Source: CAD feature listing. Evaluate the final solid. Frame: model axes, mm. Face numbers are marked on the shaded views. A direction names the side the tool comes from. Coordinates: 2 decimals unless noted, no trailing zeros. Write each loop counter-clockwise with the first axis right and the second up, starting at its lowest first coordinate (ties: lowest second). Pieces come first, ordered by that corner, then holes. Notation, with made-up numbers: (69, -8.75) -> (96, -8.75) arc R25 cw to (96, 22.25) -> close; hole circle Ø8 at (-25.5, 53). An arc over 180 degrees is marked (long way). Write item = value, one per line.
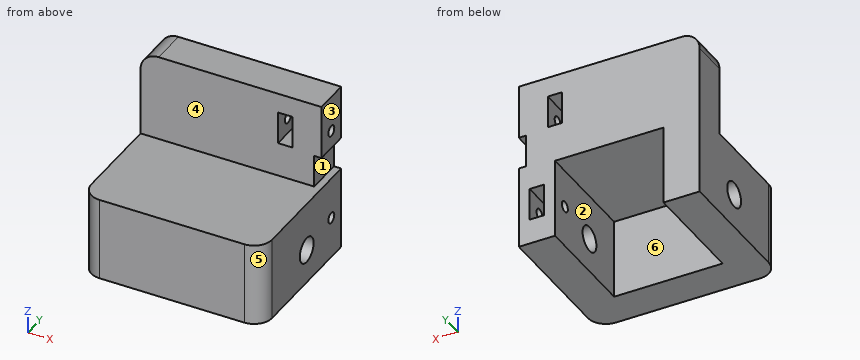
from build123d import *

# Parameters (mm, degrees)
BOSS_EXTRUDE1_DEPTH = 22
SKETCH3_W           = 10
SKETCH3_H           = 10
BOSS_EXTRUDE2_DEPTH = 25
SKETCH4_W           = 25
SKETCH4_H           = 10
BOSS_EXTRUDE3_DEPTH = 40
SKETCH5_W           = 2
SKETCH5_H           = 10
CUT_EXTRUDE4_DEPTH  = 40
BOSS_EXTRUDE4_DEPTH = 1
SKETCH7_R           = 1.5
CUT_EXTRUDE5_DEPTH  = 15
SKETCH8_W           = 4
SKETCH8_H           = 9
CUT_EXTRUDE6_DEPTH  = 15
FILLET1_R           = 5
FILLET2_R           = 5
FILLET3_R           = 5
SKETCH9_R           = 3.5
CUT_EXTRUDE7_DEPTH  = 1000
SKETCH10_W          = 4
SKETCH10_H          = 9
BOSS_EXTRUDE5_DEPTH = 15
SKETCH11_R          = 1.5
BOSS_EXTRUDE6_DEPTH = 10
SKETCH12_R          = 1.5
CUT_EXTRUDE8_DEPTH  = 19
SKETCH13_W          = 4.004831452
SKETCH13_H          = 9
CUT_EXTRUDE9_DEPTH  = 10


with BuildPart() as part:
    # Sketch1 → Boss-Extrude1 (new body)
    with BuildSketch(Plane.XY):
        Polygon((0, 30), (-10, 30), (-10, -10), (40, -10), (40, 30), (30, 30), (30, 0), (0, 0), align=None)
    extrude(amount=BOSS_EXTRUDE1_DEPTH)

    # Sketch3 → Boss-Extrude2 (add)
    with BuildSketch(Plane.XY.offset(22)):
        with Locations((-5, 25)):
            Rectangle(SKETCH3_W, SKETCH3_H)
    extrude(amount=BOSS_EXTRUDE2_DEPTH)

    # Sketch4 → Boss-Extrude3 (add)
    with BuildSketch(Plane(origin=(0, 0, 0), x_dir=(0, 0, -1), z_dir=(1, 0, 0))):
        with Locations((-34.5, 25)):
            Rectangle(SKETCH4_W, SKETCH4_H)
    extrude(amount=BOSS_EXTRUDE3_DEPTH)

    # Sketch5 → Cut-Extrude4 (cut)
    with BuildSketch(Plane.XZ.offset(-20)):
        with Locations((39, 27)):
            Rectangle(SKETCH5_W, SKETCH5_H)
    extrude(amount=-CUT_EXTRUDE4_DEPTH, mode=Mode.SUBTRACT)

    # Sketch6 → Boss-Extrude4 (add)
    with BuildSketch(Plane.XY.offset(22)):
        Polygon((-10, 20), (38, 20), (38, 30), (40, 30), (40, -10), (-10, -10), align=None)
    extrude(amount=BOSS_EXTRUDE4_DEPTH)

    # Sketch7 → Cut-Extrude5 (cut)
    with BuildSketch(Plane(origin=(40, 0, 0), x_dir=(0, 0, -1), z_dir=(1, 0, 0))):
        with Locations((-37, 25)):
            Circle(SKETCH7_R)
        with Locations((-17, 25)):
            Circle(SKETCH7_R)
    extrude(amount=-CUT_EXTRUDE5_DEPTH, mode=Mode.SUBTRACT)

    # Sketch8 → Cut-Extrude6 (cut)
    with BuildSketch(Plane(origin=(0, 30, 0), x_dir=(1, 0, 0), z_dir=(0, 1, 0))):
        with Locations((35, -17)):
            Rectangle(SKETCH8_W, SKETCH8_H)
        with Locations((30, -37)):
            Rectangle(SKETCH8_W, SKETCH8_H)
    extrude(amount=-CUT_EXTRUDE6_DEPTH, mode=Mode.SUBTRACT)

    # Fillet1
    fillet1_edges = [part.edges().sort_by_distance(p)[0] for p in [
        (40, -10, 11.5),
    ]]
    fillet(fillet1_edges, radius=FILLET1_R)

    # Fillet2
    fillet2_edges = [part.edges().sort_by_distance(p)[0] for p in [
        (-10, -10, 11.5),
    ]]
    fillet(fillet2_edges, radius=FILLET2_R)

    # Fillet3
    fillet3_edges = [part.edges().sort_by_distance(p)[0] for p in [
        (-10, 25, 47),
    ]]
    fillet(fillet3_edges, radius=FILLET3_R)

    # Sketch9 → Cut-Extrude7 (cut)
    with BuildSketch(Plane(origin=(40, 0, 0), x_dir=(0, 0, -1), z_dir=(1, 0, 0))):
        with Locations((-9.5, 12.5)):
            Circle(SKETCH9_R)
    extrude(amount=-CUT_EXTRUDE7_DEPTH, mode=Mode.SUBTRACT)

    # Sketch10 → Boss-Extrude5 (add)
    with BuildSketch(Plane(origin=(0, 30, 0), x_dir=(1, 0, 0), z_dir=(0, 1, 0))):
        with Locations((35, -17)):
            Rectangle(SKETCH10_W, SKETCH10_H)
    extrude(amount=-BOSS_EXTRUDE5_DEPTH)

    # Sketch11 → Boss-Extrude6 (add)
    with BuildSketch(Plane(origin=(40, 0, 0), x_dir=(0, 0, -1), z_dir=(1, 0, 0))):
        with Locations((-17, 25)):
            Circle(SKETCH11_R)
    extrude(amount=-BOSS_EXTRUDE6_DEPTH)

    # Sketch12 → Cut-Extrude8 (cut)
    with BuildSketch(Plane(origin=(40, 0, 0), x_dir=(0, 0, -1), z_dir=(1, 0, 0))):
        with Locations((-11.5, 25)):
            Circle(SKETCH12_R)
    extrude(amount=-CUT_EXTRUDE8_DEPTH, mode=Mode.SUBTRACT)

    # Sketch13 → Cut-Extrude9 (cut)
    with BuildSketch(Plane(origin=(0, 30, 0), x_dir=(1, 0, 0), z_dir=(0, 1, 0))):
        with Locations((35, -11.5)):
            Rectangle(SKETCH13_W, SKETCH13_H)
    extrude(amount=-CUT_EXTRUDE9_DEPTH, mode=Mode.SUBTRACT)


solid = part.part
1) Cut plane B-B, the plane z = 34. Output: boundary loops of the cut face in (x, y), and give its area (3 significant figures).
Answer block:
outline = (-10, 20) -> (28, 20) -> (28, 30) -> (-10, 30) -> close; (32, 20) -> (40, 20) -> (40, 30) -> (32, 30) -> close
area = 460 mm2
2) First-contact query: pin 1 Ø12 at (x, z) = (9, 34.5) entering from -Y; pin 2 Ø8 at (x, y) = (29.5, 6.5) entering from +Z; pin 3 Ø0.9 at (y, z) = (25.5, 37.5) entering from +X. Flat tips, straight axial feed; report the tip coordinate or a pass-through.
Answer block:
pin_1 = 20
pin_2 = 23
pin_3 = 25
3) Material intervals for probe 1 along X at (y, z) = (15, 20); probe 2 along Y at (x, z) = (34, 37); probe 3 along X at (y, z) = (26, 38.5), sorted ascending. Write a range as [from, to].
Answer block:
probe_1 = [-10, 0], [30, 40]
probe_2 = [20, 23.5], [26.5, 30]
probe_3 = [-10, 28], [32, 40]
4) Cut plane A-A, the plane y = 12.5. Output: boundary loops of the cut face in (x, z), and give its area (3 significant figures).
Answer block:
outline = (-10, 0) -> (0, 0) -> (0, 6) -> (-10, 6) -> close; (-10, 13) -> (0, 13) -> (0, 22) -> (30, 22) -> (30, 13) -> (40, 13) -> (40, 23) -> (-10, 23) -> close; (30, 0) -> (40, 0) -> (40, 6) -> (30, 6) -> close
area = 350 mm2
5) Cut plane C-C, the plane x = -2.5. Output: boundary loops of the cut face in (y, z), and give its area (3 significant figures).
Answer block:
outline = (-10, 0) -> (30, 0) -> (30, 47) -> (20, 47) -> (20, 23) -> (-10, 23) -> close; hole circle Ø7 at (12.5, 9.5)
area = 1,120 mm2
6) Reachability of the marked faces 1, 2 and 3 from +Z, -Z, +X, -X, +Y, -Y: full face, straight path, thin tool, end or side. Return the list, or none.
Answer block:
face_1 = +X, +Y, -Y
face_2 = -Z, +Y
face_3 = +Z, -Z, +X, +Y, -Y
7) Cut plane D-D, the plane y = 6.5. Output: boundary loops of the cut face in (x, z).
Answer block:
outline = (-10, 0) -> (0, 0) -> (0, 22) -> (30, 22) -> (30, 0) -> (40, 0) -> (40, 23) -> (-10, 23) -> close
8) Pull-direction query (X, two-part tool) for the marked faces 4, 5 and 6; classes: +X half, -X half, draft (parallel to the pull), parting line (faces both ways), or undercut.
Answer block:
face_4 = draft
face_5 = +X half
face_6 = undercut
